For this review, take the finished solid that the model builds, in its own axes (mm). Face numbers are marked on the shaded views. A direction names the side the tool comes from. Give positions to 0.01 mm unless a question says otherwise; leave off trailing zeros. Write each loop counter-clockwise with the first axis right and the second up, starting at its lowest first coordinate (ties: lowest second). Pieces come first, ordered by that corner, then holes. Notation, with made-up numbers: (82.5, 46.25) -> (120.5, 46.25) arc R23 ccw to (120.5, 70.25) -> close; hole circle Ø8 at (19, 22). An arc over 180 degrees is marked (long way). Answer as CSV lines item,"result".
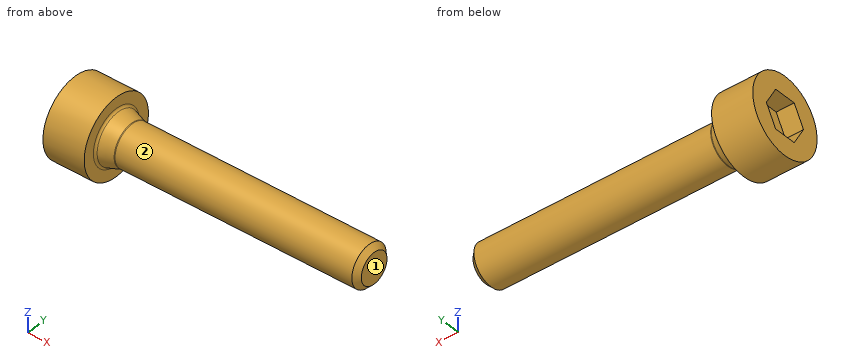
```python
from build123d import *

# Parameters (mm, degrees)
FILLET_1_R          = 0.1
CHAMFER_1_SIZE      = 0.2
CUT_EXTRUDE_1_DEPTH = 0.7


with BuildPart() as part:
    # Эскиз1 → Повернуть1 (revolve)
    with BuildSketch(Plane.XY):
        Polygon((0, 0), (0, 1.5), (1.6, 1.5), (1.6, 1), (2.2, 0.8), (11.6, 0.8), (11.6, 0), align=None)
    revolve(axis=Axis((0, 0, 0), (-1, 0, 0)))

    # Скругление1
    fillet_1_edges = [part.edges().sort_by_distance(p)[0] for p in [
        (2.2, -0.8, 0),
        (1.6, -1, 0),
    ]]
    fillet(fillet_1_edges, radius=FILLET_1_R)

    # Фаска1
    chamfer_1_edges = [part.edges().sort_by_distance(p)[0] for p in [
        (11.6, -0.8, 0),
    ]]
    chamfer(chamfer_1_edges, length=CHAMFER_1_SIZE)

    # Эскиз2 → Вырез-Вытянуть1 (cut)
    with BuildSketch(Plane.ZY):
        Polygon((0, 0.8665), (-0.750411012, 0.43325), (-0.750411012, -0.43325), (0, -0.8665), (0.750411012, -0.43325), (0.750411012, 0.43325), align=None)
    extrude(amount=-CUT_EXTRUDE_1_DEPTH, mode=Mode.SUBTRACT)


solid = part.part
```
Q1. Clearance check with flat-ended pins moving along their axes: pin 1 (0.5 mm diameter, centred on y = 0, z = 0, fed in from -X); pin 2 (1 mm diameter, centred on y = -1, z = 0.5, fed in from -X); pin 3 (1.5 mm diameter, centred on x = 3, y = 0, fed in from +Z). State where each tip first meets the part, or that it passes through.
Answer block:
pin 1,"stops at x = 0.7"
pin 2,"stops at x = 0"
pin 3,"stops at z = 0.8"
Q2. Add section A-A (y = 1.2). Write out the cut boundary in (x, z), plus the area to 3 significant figures.
Answer block:
outline,"(0, -0.9) -> (1.6, -0.9) -> (1.6, 0.9) -> (0, 0.9) -> close"
area,"2.88 mm2"
Q3. For the marked faces 1 and 2, list the 3-axis set-ups (+Z, -Z, +X, -X, +Y, -Y) from which the entire face can be reached by the end or side of a thin tool; tool diameter is ignored.
Answer block:
face 1,"+Z, -Z, +X, +Y, -Y"
face 2,"+X"
Q4. To check wall thickness, follow probe 1 along Y at (x, z) = (6.5, 0.05); probe 2 along X at (y, z) = (-1.25, 0); probe 3 along Z at (x, y) = (0.5, -0.75). State the ranges of each line that lie inside material, in increasing order. Write a range as [from, to].
Answer block:
probe 1,"y = [-0.8, 0.8]"
probe 2,"x = [0, 1.6]"
probe 3,"z = [-1.3, -0.2], [0.2, 1.3]"
